from build123d import *

# Parameters (mm, degrees)
EXTRUDE_1_DEPTH     = 14
EXTRUDE_2_DEPTH     = 3
CUT_EXTRUDE_1_DEPTH = 5
SKETCH_4_W          = 2.5
SKETCH_4_H          = 8
EXTRUDE_3_DEPTH     = 2.5


with BuildPart() as part:
    # Эскиз1 → Бобышка-Вытянуть1 (new body, symmetric)
    with BuildSketch(Plane.XY):
        Polygon((0, 35), (0, 0), (35, 0), (35, 4), (4, 4), (4, 35), align=None)
    extrude(amount=EXTRUDE_1_DEPTH, both=True)

    # Эскиз2 → Бобышка-Вытянуть2 (add)
    with BuildSketch(Plane.XY.offset(14)):
        Polygon((4, 35), (35, 4), (4, 4), align=None)
    extrude_2 = extrude(amount=-EXTRUDE_2_DEPTH)

    # Зеркальное отражение2: Бобышка-Вытянуть2 across plane
    add(extrude_2.mirror(Plane.XY))

    # Эскиз3 → Вырез-Вытянуть1 (cut, through all)
    with BuildSketch(Plane(origin=(0, 4, 0), x_dir=(1, 0, 0), z_dir=(0, 1, 0))):
        with BuildLine():
            Line((12, 3.4), (23, 3.4))
            ThreePointArc((23, 3.4), (26.4, 0), (23, -3.4))
            Line((23, -3.4), (12, -3.4))
            ThreePointArc((12, -3.4), (8.6, 0), (12, 3.4))
        make_face()
    cut_extrude_1 = extrude(amount=-CUT_EXTRUDE_1_DEPTH, mode=Mode.SUBTRACT)

    # Эскиз4 → Бобышка-Вытянуть3 (add)
    with BuildSketch(Plane.XZ):
        with Locations((4.25, 0)):
            Rectangle(SKETCH_4_W, SKETCH_4_H)
        with Locations((30.75, 0)):
            Rectangle(SKETCH_4_W, SKETCH_4_H)
    extrude_3 = extrude(amount=EXTRUDE_3_DEPTH)

    # Зеркальное отражение3: Вырез-Вытянуть1, Бобышка-Вытянуть3 across plane
    add(cut_extrude_1.mirror(Plane(origin=(0, 0, 0), x_dir=(0, 0, 1), z_dir=(-0.707106781, 0.707106781, 0))), mode=Mode.SUBTRACT)
    add(extrude_3.mirror(Plane(origin=(0, 0, 0), x_dir=(0, 0, 1), z_dir=(-0.707106781, 0.707106781, 0))))


solid = part.part
Could you check a few things on this model? Use its own coordinates, in mm. A direction names the side the tool comes from. Give positions to 0.01 mm unless a question says otherwise; leave off trailing zeros. Order: outer loops, then holes, each group sorted by start corner. A loop starts at its lowest first (then second) coordinate and runs counter-clockwise, first axis right, second up.
1. Will these pins go through, and if not, where does the flat tip stop? P1, Ø3, axis at x = 25.5, z = -0.5, coming from the -Y side; P2, Ø0.8, axis at x = -1, y = 30.5, coming from the -Z side; P3, Ø1.2, axis at x = -2, z = 0.5, coming from the +Y side; P4, Ø2, axis at x = 24.5, z = -1.5, coming from the +Y side.
2. I need wall thicknesses on L1, parallel to Z at x = 8.5, y = 11.5; L2, parallel to X at y = 5, z = -1.5; L3, parallel to Y at x = 29, z = -0.5. Which ranges of each line are inside material? Lowest first, please.
3. For faces 4 (the flat face through (32, -1, 0)), 5 (the flat face through (-1, 5.5, 0)), 6 (the flat face through (18, 2, 3.4)), 7 (the flat face through (29.5, -1, 0)), 8 (the flat face through (3, -1, 0)), which set-ups out of +Z, -Z, +X, -X, +Y, -Y let a thin tool reach every point of the face, with its end or its side?
4. Suppose I cut it at A-A (x = 20). List the corners of the cut face in (y, z) for me.
5. Suppose I cut it at B-B (z = 0). Give the number of separate pieces and of enclosed holes in the cut face, plus the area to 3 significant figures.
6. Suppose I cut it at D-D (x = 8). List the corners of the cut face in (y, z) for me.
7. We'd pull the mould along Z, two halves only. Please class faces 1 (the cylindrical face through (2, 8.6, 0.1)), 2 (the flat face through (-1, 31, -4)), 3 (the flat face through (31, -2.5, 0)): pulls with the +Z half, pulls with the -Z half, needs draft (parallel to the pull), parting line crosses it, or undercut.
Solved:
1. P1: stops at y = 0
1. P2: stops at z = -4
1. P3: stops at y = 32
1. P4: passes through
2. L1: z = -14 to -11, 11 to 14
2. L2: x = -2.5 to 4
2. L3: y = 0 to 4
3. face 4: +Z, -Z, +X, -Y
3. face 5: +Z, -Z, -X
3. face 6: +Y, -Y
3. face 7: +Z, -Z, -Y
3. face 8: +Z, -Z, -X, -Y
4. outline: (0, -14) - (19, -14) - (19, -11) - (4, -11) - (4, -3.4) - (0, -3.4) - close; (0, 3.4) - (4, 3.4) - (4, 11) - (19, 11) - (19, 14) - (0, 14) - close
5. separate pieces: 3
5. enclosed holes: 0
5. area: 147 mm2
6. outline: (0, -14) - (31, -14) - (31, -11) - (4, -11) - (4, 11) - (31, 11) - (31, 14) - (0, 14) - close
7. face 1: undercut
7. face 2: pulls with the -Z half
7. face 3: needs draft
